Source: CAD feature listing. Evaluate the final solid. Frame: model axes, mm. Round coordinates to 2 decimals unless told otherwise and drop trailing zeros. Loops run counter-clockwise (first coordinate to the right, second up) from the corner with the lowest first, then second, coordinate; pieces in that order, holes last. Notation, with made-up numbers: (88, 88) - (99, 88) arc R24 cw to (99, 127) - close; hole circle Ø8 at (86, -7.5). An arc over 180 degrees is marked (long way). One line per question, with ' | ' between items. Start each with the question number.
1. Ray query, line 1 (Y direction, x = 297, z = 1.3); line 2 (X direction, y = 1, z = 1.8); line 3 (X direction, y = 17.5, z = 1.8). Return the intervals inside material, ascending.
2. Cut plane A-A (z = 2.3). State how many separate pieces and enclosed holes the cut face has, then the cut area to 3 significant figures.
3. Cut plane B-B (y = 38). Return loops of the section in (x, z).
4. Cut plane C-C (y = -25). Return loops of the section in (x, z).
5. Mould query, pull axis X, two halves, no side actions, for faces 1 (the cylindrical face through (-4.907, -0.237, 1.479)), 2 (the cylindrical face through (-43.814, 3.764, 1.479)), 3 (the flat face through (149, 5, 0)). Classes: pulls with the +X half, pulls with the -X half, needs draft (parallel to the pull), parting line crosses it, or undercut.
6. Pin query (flat end, axial travel): pin 1 (4.5 mm diameter, centred on x = 319.75, y = -18.93, fed in from +Z). Return the tip coordinate at first contact, or that it passes through.
```python
from build123d import *

# Parameters (mm, degrees)
SKETCH_1_R      = 2.6
SKETCH_1_R_2    = 5
SKETCH_1_R_3    = 22
SKETCH_1_R_4    = 2.55
EXTRUDE_1_DEPTH = 3


with BuildPart() as part:
    # 草图1 → 凸台-拉伸1 (new body)
    with BuildSketch(Plane.XY):
        with BuildLine():
            Line((-3.823548363, 44.643956065), (296.176451637, 44.643956065))
            ThreePointArc((296.176451637, 44.643956065), (336.176451637, 4.643956065), (296.176451637, -35.356043935))
            Line((296.176451637, -35.356043935), (-3.823548363, -35.356043935))
            ThreePointArc((-3.823548363, -35.356043935), (-43.823548363, 4.643956065), (-3.823548363, 44.643956065))
        make_face()
        with Locations((-3.823548363, -19.106043935)):
            Circle(SKETCH_1_R, mode=Mode.SUBTRACT)
        with Locations((15.662023222, -6.606043935)):
            Circle(SKETCH_1_R, mode=Mode.SUBTRACT)
        with Locations((-3.823548363, 4.643956065)):
            Circle(SKETCH_1_R_2, mode=Mode.SUBTRACT)
        with Locations((296.176451637, 4.643956065)):
            Circle(SKETCH_1_R_3, mode=Mode.SUBTRACT)
        with Locations((272.606451637, 28.213956065)):
            Circle(SKETCH_1_R_4, mode=Mode.SUBTRACT)
        with Locations((319.746451637, 28.213956065)):
            Circle(SKETCH_1_R_4, mode=Mode.SUBTRACT)
        with Locations((319.746451637, -18.926043935)):
            Circle(SKETCH_1_R_4, mode=Mode.SUBTRACT)
        with Locations((272.606451637, -18.926043935)):
            Circle(SKETCH_1_R_4, mode=Mode.SUBTRACT)
        with Locations((-24.391651703, 16.518956065)):
            Circle(SKETCH_1_R, mode=Mode.SUBTRACT)
        with Locations((16.744554977, 16.518956065)):
            Circle(SKETCH_1_R, mode=Mode.SUBTRACT)
        with Locations((-23.309119948, -6.606043935)):
            Circle(SKETCH_1_R, mode=Mode.SUBTRACT)
        with Locations((-3.823548363, 27.143956065)):
            Circle(SKETCH_1_R, mode=Mode.SUBTRACT)
    extrude(amount=EXTRUDE_1_DEPTH)


solid = part.part
```
Answers follow:
1) line 1: y = -35.35 to -17.34, 26.63 to 44.64 | line 2: x = -43.66 to -7.25, -0.4 to 274.48, 317.87 to 336.01 | line 3: x = -41.7 to -26.8, -21.98 to 14.34, 19.15 to 278.32, 314.03 to 334.05
2) separate pieces: 1 | enclosed holes: 12 | area: 27,200 mm2
3) outline: (-25.9, 0) - (318.25, 0) - (318.25, 3) - (-25.9, 3) - close
4) outline: (-30.68, 0) - (323.03, 0) - (323.03, 3) - (-30.68, 3) - close
5) face 1: undercut | face 2: pulls with the -X half | face 3: needs draft
6) pin 1: passes through
